CAD build for the part. Positions are in the model's coordinates, mm. A direction names the side the tool comes from. Round coordinates to 2 decimals unless told otherwise and drop trailing zeros. Order: outer loops, then holes, each group sorted by start corner. A loop starts at its lowest first (then second) coordinate and runs counter-clockwise, first axis right, second up. Notation, with made-up numbers: M 76,22.5 L 125,22.5 A21 cw 125,49.5 Z; hole C 18,-19.75 d4. An arc over 180 degrees is marked long. Answer as CSV lines item,"result". Start each with the question number.
```python
from build123d import *

# Parameters (mm, degrees)
SKETCH1_W           = 9
SKETCH1_H           = 8
BOSS_EXTRUDE1_DEPTH = 10
CUT_EXTRUDE1_DEPTH  = 1.5
CUT_EXTRUDE2_DEPTH  = 1.5
SKETCH6_W           = 6
SKETCH6_H           = 8
CUT_EXTRUDE3_DEPTH  = 1
CUT_EXTRUDE4_DEPTH  = 8
CUT_EXTRUDE5_DEPTH  = 5
CUT_EXTRUDE6_DEPTH  = 1
CUT_EXTRUDE9_DEPTH  = 2
CUT_EXTRUDE10_DEPTH = 3


with BuildPart() as part:
    # Sketch1 → Boss-Extrude1 (new body)
    with BuildSketch(Plane.XY):
        Rectangle(SKETCH1_W, SKETCH1_H)
    extrude(amount=BOSS_EXTRUDE1_DEPTH)

    # Sketch3 → Cut-Extrude1 (cut)
    with BuildSketch(Plane(origin=(4.5, 0, 0), x_dir=(0, 0, -1), z_dir=(1, 0, 0))):
        Polygon((0, 4), (0, 0), (-3, 0), (-4, -1), (-4, 4), align=None)
    extrude(amount=-CUT_EXTRUDE1_DEPTH, mode=Mode.SUBTRACT)

    # Sketch4 → Cut-Extrude2 (cut)
    with BuildSketch(Plane(origin=(3, 0, 0), x_dir=(0, 0, -1), z_dir=(1, 0, 0))):
        Polygon((0, 4), (0, 2), (-1, 2), (-4, -1), (-4, 4), align=None)
    extrude(amount=-CUT_EXTRUDE2_DEPTH, mode=Mode.SUBTRACT)

    # Sketch6 → Cut-Extrude3 (cut)
    with BuildSketch(Plane.XZ.offset(4)):
        with Locations((1.5, 6)):
            Rectangle(SKETCH6_W, SKETCH6_H)
    extrude(amount=-CUT_EXTRUDE3_DEPTH, mode=Mode.SUBTRACT)

    # Sketch7 → Cut-Extrude4 (cut, through all)
    with BuildSketch(Plane(origin=(0, -3, 0), x_dir=(-1, 0, 0), z_dir=(0, -1, 0))):
        Polygon((-0.5, -10), (-4.5, -6), (-4.5, -10), align=None)
    extrude(amount=-CUT_EXTRUDE4_DEPTH, mode=Mode.SUBTRACT)

    # Sketch8 → Cut-Extrude5 (cut)
    with BuildSketch(Plane(origin=(0, 4, 0), x_dir=(1, 0, 0), z_dir=(0, 1, 0))):
        Polygon((4.5, -4), (4.5, -6), (0.5, -10), (-2.5, -10), (-0.5, -9), (-0.5, -6), (0.5, -5), (0.5, -4), (1.5, -4), align=None)
    extrude(amount=-CUT_EXTRUDE5_DEPTH, mode=Mode.SUBTRACT)

    # Sketch9 → Cut-Extrude6 (cut)
    with BuildSketch(Plane(origin=(1.5, 0, 0), x_dir=(0, 0, -1), z_dir=(1, 0, 0))):
        Polygon((-1, 2), (-4, 2), (-4, 4), (0, 4), (0, 2), align=None)
    extrude(amount=-CUT_EXTRUDE6_DEPTH, mode=Mode.SUBTRACT)

    # Sketch10 → Cut-Extrude9 (cut)
    with BuildSketch(Plane.ZY.offset(4.5)):
        Polygon((6, 4), (8, 1), (10, 1), (10, 4), align=None)
    extrude(amount=-CUT_EXTRUDE9_DEPTH, mode=Mode.SUBTRACT)

    # Sketch12 → Cut-Extrude10 (cut)
    with BuildSketch(Plane(origin=(0, 4, 0), x_dir=(1, 0, 0), z_dir=(0, 1, 0))):
        Polygon((0.5, -5), (-1.5, -7), (-2.5, -7), (-2.5, -10), (0.5, -8.5), align=None)
    extrude(amount=-CUT_EXTRUDE10_DEPTH, mode=Mode.SUBTRACT)


solid = part.part
```
Q1. Band-saw the part on C-C, the plane y = -0.75. Write the cut outline in (x, z).
Q2. Probe line 1 along Y through (x, z) = (-0.25, 6.25); line 2 along Z through (x, y) = (2.75, 0.5); line 3 along X through (y, z) = (-3.25, 4.5). List the from-to ranges inside material, lowest first. Write a range as from..to.
Q3. Tool access for faces 1 (the flat face through (-3.5, 2.5, 7)), 2 (the flat face through (2, -1, 6)), 3 (the flat face through (-1.5, -3.5, 5.9)), 4 (the flat face through (1, 2, 2)): list every direction of +Z, -Z, +X, -X, +Y, -Y with a clear straight run to the whole face (end or side of a thin tool).
Q4. Band-saw the part on D-D, the plane z = 5.25. Write the cut outline in (x, y), then the cut area to 4 significant figures.
Q5. Drop flat-ended pins along their axis: P1, Ø1.5, axis at y = 1, z = 2, coming from the +X side; P2, Ø1.2, axis at x = 4, z = 1.5, coming from the +Y side; P3, Ø2, axis at y = 0.5, z = 8.5, coming from the +X side; P4, Ø4, axis at y = 1, z = 3, coming from the +X side. Give the stop position or say it passes through.
Q6. Band-saw the part on A-A, the plane x = -1. Write the cut outline in (y, z).
Q7. Band-saw the part on B-B, the plane z = 1.75. Write the cut outline in (x, y).
Answer:
1,outline,"M -4.5,0 L 4.5,0 L 4.5,3.75 L 1.5,3.75 L 1.5,4 L 0.5,4 L 0.5,5 L -0.5,6 L -0.5,9 L -2.5,10 L -4.5,10 Z"
2,line 1,"y = -3..-1"
2,line 2,"z = 0..2.5"
2,line 3,"x = -4.5..-1.5"
3,face 1,"+Z, -X, +Y"
3,face 2,"+Z, +X, +Y"
3,face 3,"+Z, +X, -Y"
3,face 4,"+Z, -Z, +X, +Y"
4,outline,"M -4.5,-4 L -1.5,-4 L -1.5,-3 L 4.5,-3 L 4.5,-1 L 0.25,-1 L 0.25,4 L -4.5,4 Z"
4,area,"44.75 mm^2"
5,P1,"stops at x = 3"
5,P2,"stops at y = 0"
5,P3,"stops at x = -0.5"
5,P4,"stops at x = 4.5"
6,outline,"M -4,0 L 4,0 L 4,6.5 L 1,6.5 L 1,9.25 L -1,9.25 L -1,10 L -3,10 L -3,2 L -4,2 Z"
7,outline,"M -4.5,-4 L 4.5,-4 L 4.5,0 L 3,0 L 3,1.25 L 1.5,1.25 L 1.5,2 L 0.5,2 L 0.5,4 L -4.5,4 Z"
